Could you check a few things on this drawing? It's one solid part, dimensions in mm from its lowest x, y, z. Round coordinates to 2 decimals unless told otherwise and drop trailing zeros. Write each loop counter-clockwise with the first axis right and the second up, starting at its lowest first coordinate (ties: lowest second). Pieces come first, ordered by that corner, then holes. Notation, with made-up numbers: (25, 74.5) -> (80, 74.5) arc R26 ccw to (80, 89.5) -> close; hole circle Ø9 at (19.25, 38.5). An arc over 180 degrees is marked (long way). Return JSON: item names as keys, results as strings.
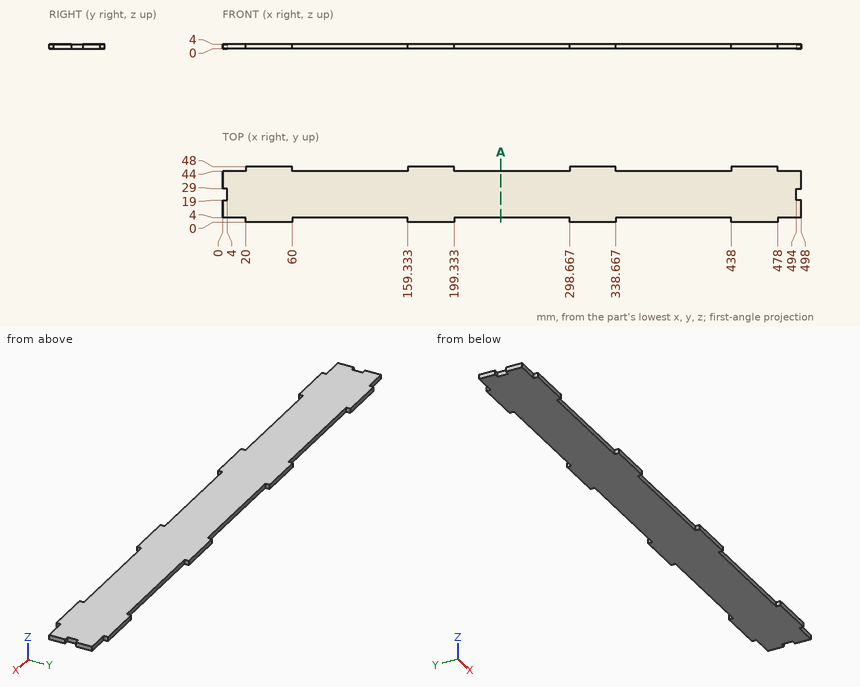
1) If I drill on probe 1 along X at (y, z) = (46, 0.6); probe 2 along X at (y, z) = (28, 1.4); probe 3 along Y at (x, z) = (393, 2.2), over which ranges is the centre line in solid material (lowest first)? Write a range as [from, to].
Return value:
{"probe 1": "[20, 60], [159.33, 199.33], [298.67, 338.67], [438, 478]", "probe 2": "[4, 494]", "probe 3": "[4, 44]"}
2) I want a section at A-A, the plane x = 239.5. Please give me the cut outline in (y, z), and give its area (3 significant figures).
Return value:
{"outline": "(4, 0) -> (44, 0) -> (44, 4) -> (4, 4) -> close", "area": "160 mm²"}
3) Will these pins go through, and if not, where does the flat tip stop? pin 1 Ø2 at (y, z) = (2.5, 2) entering from +X; pin 2 Ø2 at (x, z) = (370, 2.5) entering from +Y; pin 3 Ø2 at (y, z) = (2, 1.5) entering from -X.
Return value:
{"pin 1": "x = 478", "pin 2": "y = 44", "pin 3": "x = 20"}
